```python
from build123d import *

# Parameters (mm, degrees)
SKETCH1_R                         = 25.4
SKETCH1_R_2                       = 13.49375
BOSS_EXTRUDE1_DEPTH               = 19.05
F_10_0_1935_DIAMETER_HOLE1_REACH  = 61.906
F_10_0_1935_DIAMETER_HOLE1_BORE_R = 2.45745
CIRPATTERN1_COUNT                 = 4


with BuildPart() as part:
    # Sketch1 → Boss-Extrude1 (new body)
    with BuildSketch(Plane(origin=(0, 0, 0), x_dir=(1, 0, 0), z_dir=(0, 1, 0))):
        with Locations(Location((0, 0, 0), (0, 0, 90))):
            Circle(SKETCH1_R)
        with Locations(Location((0, 0, 0), (0, 0, 90))):
            Circle(SKETCH1_R_2, mode=Mode.SUBTRACT)
    extrude(amount=BOSS_EXTRUDE1_DEPTH)

    # #10 (0.1935) Diameter Hole1 bore → #10 (0.1935) Diameter Hole1 (cut, up to next)
    with BuildSketch(Plane(origin=(25.4, 0, 0), x_dir=(0, 0, -1), z_dir=(1, 0, 0)), mode=Mode.PRIVATE) as f_10_0_1935_diameter_hole1_sk1:
        with Locations((0, 9.525)):
            Circle(F_10_0_1935_DIAMETER_HOLE1_BORE_R)
    f_10_0_1935_diameter_hole1_tool1 = extrude(f_10_0_1935_diameter_hole1_sk1.sketch, amount=-F_10_0_1935_DIAMETER_HOLE1_REACH, mode=Mode.PRIVATE) & part.part
    f_10_0_1935_diameter_hole1 = f_10_0_1935_diameter_hole1_tool1.solids().sort_by_distance((25.4, 9.525, 0))[0]
    add(f_10_0_1935_diameter_hole1, mode=Mode.SUBTRACT)

    # CirPattern1: #10 (0.1935) Diameter Hole1 ×4 about axis
    cirpattern1_axis = Axis((0, 19.05, 0), (0, -1, 0))
    for i in range(1, CIRPATTERN1_COUNT):
        add(f_10_0_1935_diameter_hole1.rotate(cirpattern1_axis, i * 360 / CIRPATTERN1_COUNT), mode=Mode.SUBTRACT)


solid = part.part
```
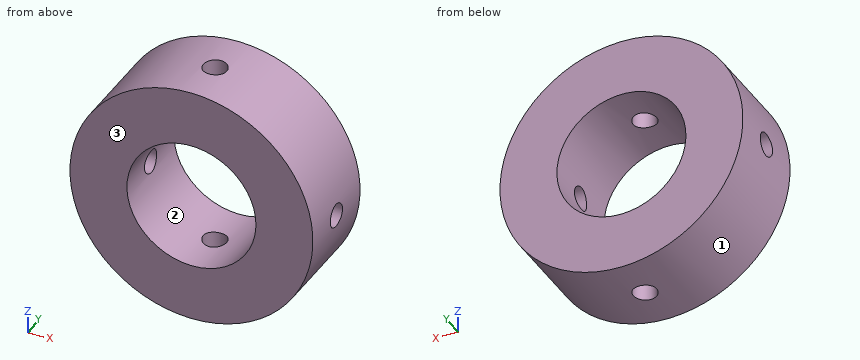
Geometry check sheet. Reference: the model listing, model coordinates, mm. Face numbers are marked on the shaded views. Give positions to 0.01 mm unless a question says otherwise; leave off trailing zeros. Write each loop counter-clockwise with the first axis right and the second up, starting at its lowest first coordinate (ties: lowest second). Pieces come first, ordered by that corner, then holes. Notation, with made-up numbers: (76.25, 89) -> (122.25, 89) arc R20 cw to (122.25, 118) -> close; hole circle Ø1 at (29, -13.5). An arc over 180 degrees is marked (long way). Use one line per item in the form item = value.
Item 1: Sectioned sample at A-A on x = 0. Enter the section's corners in (y, z), plus the area to 3 significant figures.
Results list:
outline = (0, -25.4) -> (7.07, -25.4) -> (7.07, -13.49) -> (0, -13.49) -> close; (0, 13.49) -> (7.07, 13.49) -> (7.07, 25.4) -> (0, 25.4) -> close; (11.98, -25.4) -> (19.05, -25.4) -> (19.05, -13.49) -> (11.98, -13.49) -> close; (11.98, 13.49) -> (19.05, 13.49) -> (19.05, 25.4) -> (11.98, 25.4) -> close
area = 337 mm2
Item 2: Sectioned sample at C-C on x = 9. Enter the section's corners in (y, z), plus the area to 3 significant figures.
Results list:
outline = (0, -23.75) -> (19.05, -23.75) -> (19.05, -10.05) -> (0, -10.05) -> close; (0, 10.05) -> (19.05, 10.05) -> (19.05, 23.75) -> (0, 23.75) -> close
area = 522 mm2
Item 3: Depth check by flat-ended pin: pin 1 Ø8 at (x, y) = (6.5, 9) entering from -Z; pin 2 Ø3 at (x, y) = (17, 4.5) entering from -Z; pin 3 Ø2 at (x, y) = (2.5, 5.5) entering from -Z. Enter the tip coordinate at first touch or a pass-through.
Results list:
pin_1 = -25.28
pin_2 = -20.12
pin_3 = -25.36
Item 4: Sectioned sample at D-D on z = 7. Enter the section's corners in (x, y).
Results list:
outline = (-24.42, 0) -> (-11.54, 0) -> (-11.54, 19.05) -> (-24.42, 19.05) -> close; (11.54, 0) -> (24.42, 0) -> (24.42, 19.05) -> (11.54, 19.05) -> close
Item 5: Mould release check, pull along Z, two halves, no side actions. Record for the marked faces 1, 2 and 3: released by +Z, released by -Z, zero draft, split by the parting line, or undercut.
Results list:
face_1 = split by the parting line
face_2 = undercut
face_3 = zero draft
Item 6: Sectioned sample at B-B on z = 0. Enter the section's corners in (x, y), plus the area to 3 significant figures.
Results list:
outline = (-25.4, 0) -> (-13.49, 0) -> (-13.49, 7.07) -> (-25.4, 7.07) -> close; (-25.4, 11.98) -> (-13.49, 11.98) -> (-13.49, 19.05) -> (-25.4, 19.05) -> close; (13.49, 0) -> (25.4, 0) -> (25.4, 7.07) -> (13.49, 7.07) -> close; (13.49, 11.98) -> (25.4, 11.98) -> (25.4, 19.05) -> (13.49, 19.05) -> close
area = 337 mm2
Item 7: Scan lines: line 1 (Y direction, x = 18, z = 0); line 2 (Z direction, x = 0, y = 1); line 3 (X direction, y = 8.25, z = -19.5). Record each from-to range of solid material in increasing order.
Results list:
line_1 = 0 to 7.07, 11.98 to 19.05
line_2 = -25.4 to -13.49, 13.49 to 25.4
line_3 = -16.28 to -2.1, 2.1 to 16.28
